Autodesk Inventor part; units mm, degrees
ref_plane "YZ Plane" through (0, 0, 0) normal (1, 0, 0) x (0, 1, 0)
ref_plane "XZ Plane" through (0, 0, 0) normal (0, 1, 0) x (-1, 0, 0)
ref_plane "XY Plane" through (0, 0, 0) normal (0, 0, 1) x (1, 0, 0)
sketch "Sketch1" plane through (0, 0, 0) normal (1, 0, 0) x (0, 1, 0)
  line L0 (0, 0) -> (22, 0)
  line L1 (22, 0) -> (22, -255)
  line L2 (22, -255) -> (0, -255)
  line L3 (0, -255) -> (0, 0)
  line L4 (0, -255) -> (2.8219, -233.1817)
  line L5 (2.8219, -233.1817) -> (255.7155, -265.8902)
  line L6 (255.7155, -265.8902) -> (252.8936, -287.7085)
  line L7 (252.8936, -287.7085) -> (0, -255)
  point P0 (22, -235.6622)
  dimension "d0" = 22
  dimension "d1" = 255
  dimension "d2" = 22
  dimension "d3" = 255
extrude "Extrusion1" add sketch "Sketch1" along normal blind 363.4
chamfer "Chamfer1" distance 20 angle 45 4 edges at (363.4, 254.3045, -276.7993) (0, 254.3045, -276.7993) (363.4, 11, 0) (0, 11, 0)
sketch "Sketch2" plane through (0, 22, -235.6622) normal (0, 0.1282685, 0.9917395) x (1, 0, 0)
  line L0 (8, 215.6622) -> (355.4, 215.6622)
  line L1 (355.4, 215.6622) -> (355.4, 15)
  line L2 (355.4, 15) -> (8, 15)
  line L3 (8, 15) -> (8, 215.6622)
  line L4 (0, 215.6622) -> (0, 0)
  line L5 (363.4, 215.6622) -> (363.4, 0)
  line L6 (20, 235.6622) -> (343.4, 235.6622)
  line L7 (0, 0) -> (363.4, 0)
  point P0 (0, -52.0463)
  dimension "d9" = 8
  dimension "d10" = 8
  dimension "d11" = 20
  dimension "d12" = 15
extrude "Extrusion2" cut sketch "Sketch2" against normal blind 5
sketch "Sketch4" plane through (0, 22, -235.6622) normal (0, 1, 0) x (1, 0, 0)
  line L0 (24, -24.076) -> (339.4, -24.076)
  line L1 (339.4, -24.076) -> (339.4, -131.6622)
  line L2 (339.4, -131.6622) -> (24, -131.6622)
  line L3 (24, -131.6622) -> (24, -24.076)
  line L4 (355.4, 1.924) -> (8, 1.924)
  line L5 (0, 0) -> (0, -215.6622)
  line L6 (363.4, 0) -> (363.4, -215.6622)
  line L7 (20, -235.6622) -> (343.4, -235.6622)
  dimension "d15" = 26
  dimension "d16" = 24
  dimension "d17" = 24
  dimension "d18" = 104
extrude "Extrusion3" add sketch "Sketch4" along normal blind 5
properties part number "Laptop" material "PBT Plastic"
Input: part model. Units: mm. Frame: model coordinates. A direction names the side the tool comes from. Round coordinates to 2 decimals unless told otherwise and drop trailing zeros. Order: outer loops, then holes, each group sorted by start corner. A loop starts at its lowest first (then second) coordinate and runs counter-clockwise, first axis right, second up. Notation, with made-up numbers: (-7.75, 11.25) - (30.25, 11.25) arc R17 cw to (30.25, 33.25) - close; hole circle Ø5 at (29.25, -11.75). An arc over 180 degrees is marked (long way). Answer as a JSON object with one key per item and string values. Group by question number.
(1) Cut plane D-D (z = -51.5). Return loops of the section in (x, y).
(2) Pin query (flat end, axial travel): P1, Ø3, axis at x = 116.5, y = 54, coming from the -Z side; P2, Ø4, axis at y = 25, z = -137.5, coming from the +X side; P3, Ø4, axis at x = 224, y = 25, coming from the -Z side. Return the tip coordinate at first contact, or that it passes through.
(3) Material intervals for probe 1 along X at (y, z) = (25, -107.5); probe 2 along Y at (x, z) = (286, -187); probe 3 along Y at (x, z) = (161, -70.5), sorted ascending. Write a range as from..to.
(4) Reachability of faces 1 (the face through (353.26, 244.546, -275.382)), 2 (the face through (180.85, 34.44, -237.27)), 3 (the face through (179, 27, -159)) from +Z, -Z, +X, -X, +Y, -Y: full face, straight path, thin tool, end or side. Return the list, or none.
(5) Draft query along Z for faces 4 (the face through (353.5, 11.2, -10.1)), 5 (the face through (363.4, 21, -201)), 6 (the face through (179, 22, -90)). Return one class per face: released by +Z, released by -Z, zero draft, split by the parting line, or undercut.
(6) Cut plane C-C (y = 165.5). Return loops of the section in (x, z).
(7) Cut plane B-B (x = 204.5). Return loops of the section in (y, z).
(8) Cut plane A-A (z = -174). Return loops of the section in (x, y).
Here are the results:
{
 "1": {"outline": "(0, 0) - (363.4, 0) - (363.4, 22) - (0, 22) - close"},
 "2": {"P1": "stops at z = -262.18", "P2": "stops at x = 339.4", "P3": "stops at z = -258.49"},
 "3": {"probe 1": "x = 24..339.4", "probe 2": "y = 0..27", "probe 3": "y = 0..22"},
 "4": {"face 1": "-Z, +X, +Y", "face 2": "+X, -X, +Y", "face 3": "+Z, +X, -X, +Y"},
 "5": {"face 4": "released by +Z", "face 5": "zero draft", "face 6": "undercut"},
 "6": {"outline": "(0, -276.41) - (363.4, -276.41) - (363.4, -254.22) - (355.4, -254.22) - (355.4, -259.27) - (8, -259.27) - (8, -254.22) - (0, -254.22) - close"},
 "7": {"outline": "(0, -255) - (252.89, -287.71) - (255.72, -265.89) - (235.88, -263.32) - (235.24, -268.29) - (36.23, -242.55) - (36.88, -237.59) - (22, -235.66) - (22, -211.59) - (27, -211.59) - (27, -104) - (22, -104) - (22, 0) - (0, 0) - close"},
 "8": {"outline": "(0, 0) - (363.4, 0) - (363.4, 22) - (339.4, 22) - (339.4, 27) - (24, 27) - (24, 22) - (0, 22) - close"}
}
